from build123d import *

# Parameters (mm, degrees)
BOSS_EXTRUDE1_DEPTH = 127
SKETCH2_R           = 2.1828125
CUT_EXTRUDE1_DEPTH  = 127


with BuildPart() as part:
    # Sketch1 → Boss-Extrude1 (new body)
    with BuildSketch(Plane.XY):
        Polygon((0, 0), (0, 38.1), (1.5875, 38.1), (1.5875, 1.5875), (38.1, 1.5875), (38.1, 0), align=None)
    extrude(amount=BOSS_EXTRUDE1_DEPTH)

    # Sketch2 → Cut-Extrude1 (cut)
    with BuildSketch(Plane(origin=(0, 1.5875, 0), x_dir=(1, 0, 0), z_dir=(0, 1, 0))):
        with Locations(Location((23.1775, -114.3, 0), (0, 0, 180))):
            Circle(SKETCH2_R)
        with Locations(Location((23.1775, -101.6, 0), (0, 0, 180))):
            Circle(SKETCH2_R)
        with Locations(Location((23.1775, -88.9, 0), (0, 0, 180))):
            Circle(SKETCH2_R)
        with Locations(Location((23.1775, -76.2, 0), (0, 0, 180))):
            Circle(SKETCH2_R)
        with Locations(Location((23.1775, -63.5, 0), (0, 0, 180))):
            Circle(SKETCH2_R)
        with Locations(Location((23.1775, -50.8, 0), (0, 0, 180))):
            Circle(SKETCH2_R)
    extrude(amount=-CUT_EXTRUDE1_DEPTH, mode=Mode.SUBTRACT)


solid = part.part
For this review, take the finished solid that the model builds, in its own axes (mm). A direction names the side the tool comes from. Round coordinates to 2 decimals unless told otherwise and drop trailing zeros. Order: outer loops, then holes, each group sorted by start corner. A loop starts at its lowest first (then second) coordinate and runs counter-clockwise, first axis right, second up. Notation, with made-up numbers: M 31.5,-26 L 47.5,-26 A17 cw 47.5,-1 Z; hole C 67.5,57.5 d7. An arc over 180 degrees is marked long. Use a Markdown table: item, result. Add a question column.
Item 1: Tool access review of faces 1 (the flat face through (1.588, 20, 63)), 2 (the cylindrical face through (23.462, 0.805, 116.464)): name each direction out of +Z, -Z, +X, -X, +Y, -Y from which nothing blocks a thin tool from reaching the whole face with its end or side.
Item 2: Mouldability with a two-part tool opening along X and no side actions: class faces 3 (the flat face through (19, 0, 63)), 4 (the cylindrical face through (23.462, 0.805, 103.764)), 5 (the flat face through (0, 19, 63)) as released by +X, released by -X, zero draft, split by the parting line, or undercut.
Item 3: Add section A-A, the plane z = 88.9. Give the boundary of the cut face in (x, y), then the cut area to 3 significant figures.
Item 4: Add section C-C, the plane x = 19. Give the boundary of the cut face in (y, z).
Item 5: Add section B-B, the plane z = 42. Give the boundary of the cut face in (x, y), then the cut area to 3 significant figures.
Item 6: To check wall thickness, follow line 1 along X through (y, z) = (36.5, 80.5). State the ranges of the line that lie inside material, in increasing order.
Item 7: Insertion check: pin 1 (11 mm diameter, centred on y = 20, z = 57, fed in from +X); pin 2 (5.5 mm diameter, centred on x = 23.18, z = 88.9, fed in from +Y). Each pin has a flat end and moves straight along its axis. Give the tip position at first contact, or say it passes through.
Geometry results:
| question | item | result |
|---|---|---|
| 1 | face 1 | +Z, -Z, +X, +Y |
| 1 | face 2 | +Y, -Y |
| 2 | face 3 | zero draft |
| 2 | face 4 | undercut |
| 2 | face 5 | released by -X |
| 3 | outline | M 0,0 L 20.99,0 L 20.99,1.59 L 1.59,1.59 L 1.59,38.1 L 0,38.1 Z; M 25.36,0 L 38.1,0 L 38.1,1.59 L 25.36,1.59 Z |
| 3 | area | 112 mm² |
| 4 | outline | M 0,0 L 1.59,0 L 1.59,127 L 0,127 Z |
| 5 | outline | M 0,0 L 38.1,0 L 38.1,1.59 L 1.59,1.59 L 1.59,38.1 L 0,38.1 Z |
| 5 | area | 118 mm² |
| 6 | line 1 | x = 0 to 1.59 |
| 7 | pin 1 | stops at x = 1.59 |
| 7 | pin 2 | stops at y = 1.59 |
